Check sheet for the modelled part. Datum: model origin and axes. Units: mm. A direction names the side the tool comes from. Round coordinates to 2 decimals unless told otherwise and drop trailing zeros. Write each loop counter-clockwise with the first axis right and the second up, starting at its lowest first coordinate (ties: lowest second). Pieces come first, ordered by that corner, then holes. Notation, with made-up numbers: (56.25, 63.25) - (100.25, 63.25) arc R18 cw to (100.25, 91.25) - close; hole circle Ø6 at (-3, -40). An arc over 180 degrees is marked (long way). Use one line per item in the form item = value. Start each with the question number.
1) Section check B-B (z = 219). Record the boundary of the cut face in (x, y), then the cut area to 3 significant figures.
2) Scan lines: probe 1 along Y at (x, z) = (0.65, 292); probe 2 along Y at (x, z) = (9.7, 247.1); probe 3 along X at (y, z) = (20.5, 227). Record each from-to range of solid material in increasing order.
3) Set-up check for faces 1 (the face through (9, 20, 163)), 2 (the face through (5, 40, 163)): record each of +Z, -Z, +X, -X, +Y, -Y from which the full face is reachable in a straight line by a thin tool's end or side.
4) Section check A-A (y = 30.5). Record the boundary of the cut face in (x, z), then the cut area to 3 significant figures.
5) Draft check along X on faces 3 (the face through (0, 20, 163)), 4 (the face through (0.5, 21.6, 0)), 5 (the face through (1, 20, 163)). Enter one of: +X half, -X half, draft (parallel to the pull), parting line (faces both ways), or undercut.
from build123d import *

# Parameters (mm, degrees)
SKETCH_1_W               = 10
SKETCH_1_H               = 40
SKETCH_1_W_2             = 8
SKETCH_1_H_2             = 38
EXTRUDE_1_DEPTH          = 330
SKETCH_3_R               = 1.5
CUT_EXTRUDE_2_DEPTH      = 10
CUT_EXTRUDE_4_DEPTH      = 333.565782966
CUT_EXTRUDE_4_DEPTH_BACK = 333.565782966
SKETCH_4_R               = 2


with BuildPart() as part:
    # 草图1 → 凸台-拉伸1 (new body)
    with BuildSketch(Plane.XY):
        with Locations((5, 20)):
            Rectangle(SKETCH_1_W, SKETCH_1_H)
        with Locations((5, 20)):
            Rectangle(SKETCH_1_W_2, SKETCH_1_H_2, mode=Mode.SUBTRACT)
    extrude(amount=EXTRUDE_1_DEPTH)

    # 草图3 → 切除-拉伸2 (cut)
    with BuildSketch(Plane(origin=(10, 0, 0), x_dir=(0, 0, -1), z_dir=(1, 0, 0))):
        with Locations((-308, 18.5)):
            Circle(SKETCH_3_R)
        with Locations((-292, 18.5)):
            Circle(SKETCH_3_R)
        with Locations((-292, 3.5)):
            Circle(SKETCH_3_R)
        with Locations((-308, 3.5)):
            Circle(SKETCH_3_R)
        with Locations((-263.1, 36.5)):
            Circle(SKETCH_3_R)
        with Locations((-247.1, 36.5)):
            Circle(SKETCH_3_R)
        with Locations((-263.1, 21.5)):
            Circle(SKETCH_3_R)
        with Locations((-247.1, 21.5)):
            Circle(SKETCH_3_R)
    extrude(amount=-CUT_EXTRUDE_2_DEPTH, mode=Mode.SUBTRACT)

    # 草图4 → 切除-拉伸4 (cut, two sides: drawn at the far end of the back side and taken through both)
    with BuildSketch(Plane(origin=(0, 40, 0), x_dir=(1, 0, 0), z_dir=(0, 1, 0)).offset(-CUT_EXTRUDE_4_DEPTH_BACK)):
        with Locations(Location((5, -10, 0), (0, 0, 90))):
            Circle(SKETCH_4_R)
        with Locations(Location((5, -20, 0), (0, 0, 90))):
            Circle(SKETCH_4_R)
        with Locations(Location((5, -30, 0), (0, 0, 90))):
            Circle(SKETCH_4_R)
        with Locations(Location((5, -40, 0), (0, 0, 90))):
            Circle(SKETCH_4_R)
    extrude(amount=CUT_EXTRUDE_4_DEPTH + CUT_EXTRUDE_4_DEPTH_BACK, mode=Mode.SUBTRACT)


solid = part.part
Results are:
q1.outline = (0, 0) - (10, 0) - (10, 40) - (0, 40) - close; hole (1, 1) - (9, 1) - (9, 39) - (1, 39) - close
q1.area = 96.0 mm²
q2.probe_1 = 0 to 2, 5 to 17, 20 to 40
q2.probe_2 = 0 to 20, 23 to 35, 38 to 40
q2.probe_3 = 0 to 1, 9 to 10
q3.face_1 = +Z, -Z
q3.face_2 = +Z, -Z, +X, -X, +Y
q4.outline = (0, 0) - (1, 0) - (1, 330) - (0, 330) - close; (9, 0) - (10, 0) - (10, 330) - (9, 330) - close
q4.area = 660 mm²
q5.face_3 = -X half
q5.face_4 = draft
q5.face_5 = undercut
